The listing builds one solid part. Answer for the finished solid, in the listing's coordinates (mm). Coordinates: 2 decimals unless noted, no trailing zeros. Write each loop counter-clockwise with the first axis right and the second up, starting at its lowest first coordinate (ties: lowest second). Pieces come first, ordered by that corner, then holes.
from build123d import *

# Parameters (mm, degrees)
BOSS_EXTRUDE1_DEPTH     = 3
M3_CLEARANCE_HOLE1_D    = 3.4
BOSS_EXTRUDE3_START     = -3
SKETCH31_R              = 1.7
BOSS_EXTRUDE3_DEPTH     = 3
CUT_EXTRUDE5_DEPTH      = 10
CUT_EXTRUDE6_DEPTH      = 227.875050806
CUT_EXTRUDE6_DEPTH_BACK = 227.875050806
SKETCH32_R              = 1.7
SKETCH32_W              = 8
SKETCH32_H              = 29.5
FILLET4_R               = 2


with BuildPart() as part:
    # Sketch1 → Boss-Extrude1 (new body)
    with BuildSketch(Plane(origin=(0, 0, 0), x_dir=(1, 0, 0), z_dir=(0, 1, 0))):
        with BuildLine():
            Line((-135.5, 14.75), (135.5, 14.75))
            ThreePointArc((135.5, 14.75), (137.267766953, 14.017766953), (138, 12.25))
            Line((138, 12.25), (138, -12.25))
            ThreePointArc((138, -12.25), (137.267766953, -14.017766953), (135.5, -14.75))
            Line((135.5, -14.75), (-135.5, -14.75))
            ThreePointArc((-135.5, -14.75), (-137.267766953, -14.017766953), (-138, -12.25))
            Line((-138, -12.25), (-138, 12.25))
            ThreePointArc((-138, 12.25), (-137.267766953, 14.017766953), (-135.5, 14.75))
        make_face()
    extrude(amount=BOSS_EXTRUDE1_DEPTH)

    # M3 Clearance Hole1 (through all)
    with Locations(Plane.XZ):
        with Locations((-133.5, 12.25), (-126.5, 12.25), (-133.5, -12.25), (-126.5, -12.25), (-68.5, 12.25), (-61.5, 12.25), (-68.5, -12.25), (-61.5, -12.25), (-3.5, 12.25), (3.5, 12.25), (-3.5, -12.25), (3.5, -12.25), (61.5, 12.25), (68.5, 12.25), (61.5, -12.25), (68.5, -12.25), (126.5, 12.25), (133.5, 12.25), (126.5, -12.25), (133.5, -12.25), (94, -12.25), (101, -12.25)):
            Hole(M3_CLEARANCE_HOLE1_D / 2)

    # Sketch31 → Boss-Extrude3 (add)
    with BuildSketch(Plane(origin=(0, 3, 0), x_dir=(1, 0, 0), z_dir=(0, 1, 0)).offset(BOSS_EXTRUDE3_START)):
        with BuildLine():
            Line((135.5, 14.75), (183.187594482, 14.75))
            ThreePointArc((183.187594482, 14.75), (183.527894438, 14.726730898), (183.861859615, 14.657356752))
            Line((183.861859615, 14.657356752), (224.91460107, 3.159089135))
            ThreePointArc((224.91460107, 3.159089135), (225.968742259, 2.441751578), (226.375188963, 1.233203733))
            Line((226.375188963, 1.233203733), (226.375188963, -12.75))
            ThreePointArc((226.375188963, -12.75), (225.789402526, -14.164213562), (224.375188963, -14.75))
            Line((224.375188963, -14.75), (135.5, -14.75))
            ThreePointArc((135.5, -14.75), (137.267766953, -14.017766953), (138, -12.25))
            Line((138, -12.25), (138, 12.25))
            ThreePointArc((138, 12.25), (137.267766953, 14.017766953), (135.5, 14.75))
        make_face()
        with Locations(Location((171.687594482, 12.25, 0), (0, 0, 270))):
            Circle(SKETCH31_R, mode=Mode.SUBTRACT)
        with Locations(Location((178.687594482, 12.25, 0), (0, 0, 270))):
            Circle(SKETCH31_R, mode=Mode.SUBTRACT)
        with Locations(Location((178.687594482, -12.25, 0), (0, 0, 90))):
            Circle(SKETCH31_R, mode=Mode.SUBTRACT)
        with Locations(Location((171.687594482, -12.25, 0), (0, 0, 90))):
            Circle(SKETCH31_R, mode=Mode.SUBTRACT)
    extrude(amount=BOSS_EXTRUDE3_DEPTH)

    # Sketch29 → Cut-Extrude5 (cut)
    with BuildSketch(Plane.XZ):
        with BuildLine():
            Line((-80.5, 5.3456), (-80.5, -1.4522))
            ThreePointArc((-80.5, -1.4522), (-81.085786438, -2.866413562), (-82.5, -3.4522))
            Line((-82.5, -3.4522), (-138, -3.4522))
            Line((-138, -3.4522), (-138, 9.8456))
            ThreePointArc((-138, 9.8456), (-137.267766953, 8.077833047), (-135.5, 7.3456))
            Line((-135.5, 7.3456), (-82.5, 7.3456))
            ThreePointArc((-82.5, 7.3456), (-81.085786438, 6.759813562), (-80.5, 5.3456))
        make_face()
    extrude(amount=-CUT_EXTRUDE5_DEPTH, mode=Mode.SUBTRACT)

    # Sketch32 → Cut-Extrude6 (cut, two sides: drawn at the far end of the back side and taken through both)
    with BuildSketch(Plane(origin=(0, 0, 0), x_dir=(1, 0, 0), z_dir=(0, 1, 0)).offset(-CUT_EXTRUDE6_DEPTH_BACK)):
        with Locations(Location((-119.5, 12.25, 0), (0, 0, 270))):
            Circle(SKETCH32_R)
        with Locations(Location((-119.5, -12.25, 0), (0, 0, 270))):
            Circle(SKETCH32_R)
        with Locations((-134, 0)):
            Rectangle(SKETCH32_W, SKETCH32_H)
    extrude(amount=CUT_EXTRUDE6_DEPTH + CUT_EXTRUDE6_DEPTH_BACK, mode=Mode.SUBTRACT)

    # Fillet4
    fillet4_edges = [part.edges().sort_by_distance(p)[0] for p in [
        (-130, 1.5, -3.4522),
        (-130, 1.5, 14.75),
        (-130, 1.5, 7.3456),
        (-130, 1.5, -14.75),
    ]]
    fillet(fillet4_edges, radius=FILLET4_R)


solid = part.part
1. Find the intervals of material crossed by L1, parallel to Z at x = 133.5, y = 0.9; L2, parallel to Z at x = 2, y = 1.65; L3, parallel to X at y = 1.75, z = 9.25, in increasing order.
Results found:
L1: z = -14.75 to -13.95, -10.55 to 10.55, 13.95 to 14.75
L2: z = -14.75 to -13.05, -11.45 to 11.45, 13.05 to 14.75
L3: x = -130 to 226.38
2. Flat-ended cylindrical pins translate along their axes: P1, Ø2.5, axis at x = 61.5, z = -12.25, coming from the +Y side; P2, Ø0.9, axis at y = 2, z = 3.5, coming from the -X side. Find the tip coordinate at first contact, or state that the pin passes through.
Results found:
P1: passes through
P2: stops at x = -80.5
3. Section B-B on x = 187.5 is taken. Give the vertices of the cut face in (y, z).
Results found:
outline: (0, -13.64) - (3, -13.64) - (3, 14.75) - (0, 14.75) - close
4. Section A-A on y = 1.4 is taken. State how many separate pieces and enclosed holes the cut face has, then the cut area to 3 significant figures.
Results found:
separate pieces: 1
enclosed holes: 26
area: 9,480 mm2
